Source: CAD feature listing. Evaluate the final solid. Frame: model axes, mm. Round coordinates to 2 decimals unless told otherwise and drop trailing zeros. Write each loop counter-clockwise with the first axis right and the second up, starting at its lowest first coordinate (ties: lowest second). Pieces come first, ordered by that corner, then holes.
from build123d import *

# Parameters (mm, degrees)
BOSS_EXTRUDE1_DEPTH = 5
FILLET1_R           = 8
SKETCH2_R           = 12.5
CUT_EXTRUDE1_DEPTH  = 10


with BuildPart() as part:
    # Sketch1 → Boss-Extrude1 (new body)
    with BuildSketch(Plane(origin=(0, 0, 0), x_dir=(1, 0, 0), z_dir=(0, 1, 0))):
        Polygon((-75.055534995, 0), (-37.527767497, -65), (37.527767497, -65), (75.055534995, 0), (37.527767497, 65), (-37.527767497, 65), align=None)
    extrude(amount=BOSS_EXTRUDE1_DEPTH)

    # Fillet1
    fillet1_edges = [part.edges().sort_by_distance(p)[0] for p in [
        (-37.527767497, 2.5, -65),
        (37.527767497, 2.5, -65),
        (75.055534995, 2.5, 0),
        (37.527767497, 2.5, 65),
        (-37.527767497, 2.5, 65),
        (-75.055534995, 2.5, 0),
    ]]
    fillet(fillet1_edges, radius=FILLET1_R)

    # Sketch2 → Cut-Extrude1 (cut)
    with BuildSketch(Plane(origin=(0, 5, 0), x_dir=(1, 0, 0), z_dir=(0, 1, 0))):
        with Locations(Location((0, 0, 0), (0, 0, 270))):
            Circle(SKETCH2_R)
        with BuildLine():
            Line((9.526279442, 26.5), (24.248711306, 52))
            ThreePointArc((24.248711306, 52), (24.248711306, 54), (22.516660498, 55))
            Line((22.516660498, 55), (-22.516660498, 55))
            ThreePointArc((-22.516660498, 55), (-24.248711306, 54), (-24.248711306, 52))
            Line((-24.248711306, 52), (-9.526279442, 26.5))
            ThreePointArc((-9.526279442, 26.5), (-8.42820323, 25.401923789), (-6.92820323, 25))
            Line((-6.92820323, 25), (6.92820323, 25))
            ThreePointArc((6.92820323, 25), (8.42820323, 25.401923789), (9.526279442, 26.5))
        make_face()
        with BuildLine():
            Line((27.712812921, 5), (57.15767665, 5))
            ThreePointArc((57.15767665, 5), (58.889727457, 6), (58.889727457, 8))
            Line((58.889727457, 8), (36.373066959, 47))
            ThreePointArc((36.373066959, 47), (34.641016151, 48), (32.908965344, 47))
            Line((32.908965344, 47), (18.186533479, 21.5))
            ThreePointArc((18.186533479, 21.5), (17.784609691, 20), (18.186533479, 18.5))
            Line((18.186533479, 18.5), (25.11473671, 6.5))
            ThreePointArc((25.11473671, 6.5), (26.212812921, 5.401923789), (27.712812921, 5))
        make_face()
        with BuildLine():
            Line((18.186533479, -21.5), (32.908965344, -47))
            ThreePointArc((32.908965344, -47), (34.641016151, -48), (36.373066959, -47))
            Line((36.373066959, -47), (58.889727457, -8))
            ThreePointArc((58.889727457, -8), (58.889727457, -6), (57.15767665, -5))
            Line((57.15767665, -5), (27.712812921, -5))
            ThreePointArc((27.712812921, -5), (26.212812921, -5.401923789), (25.11473671, -6.5))
            Line((25.11473671, -6.5), (18.186533479, -18.5))
            ThreePointArc((18.186533479, -18.5), (17.784609691, -20), (18.186533479, -21.5))
        make_face()
        with BuildLine():
            Line((-9.526279442, -26.5), (-24.248711306, -52))
            ThreePointArc((-24.248711306, -52), (-24.248711306, -54), (-22.516660498, -55))
            Line((-22.516660498, -55), (22.516660498, -55))
            ThreePointArc((22.516660498, -55), (24.248711306, -54), (24.248711306, -52))
            Line((24.248711306, -52), (9.526279442, -26.5))
            ThreePointArc((9.526279442, -26.5), (8.42820323, -25.401923789), (6.92820323, -25))
            Line((6.92820323, -25), (-6.92820323, -25))
            ThreePointArc((-6.92820323, -25), (-8.42820323, -25.401923789), (-9.526279442, -26.5))
        make_face()
        with BuildLine():
            Line((-27.712812921, -5), (-57.15767665, -5))
            ThreePointArc((-57.15767665, -5), (-58.889727457, -6), (-58.889727457, -8))
            Line((-58.889727457, -8), (-36.373066959, -47))
            ThreePointArc((-36.373066959, -47), (-34.641016151, -48), (-32.908965344, -47))
            Line((-32.908965344, -47), (-18.186533479, -21.5))
            ThreePointArc((-18.186533479, -21.5), (-17.784609691, -20), (-18.186533479, -18.5))
            Line((-18.186533479, -18.5), (-25.11473671, -6.5))
            ThreePointArc((-25.11473671, -6.5), (-26.212812921, -5.401923789), (-27.712812921, -5))
        make_face()
        with BuildLine():
            Line((-18.186533479, 21.5), (-32.908965344, 47))
            ThreePointArc((-32.908965344, 47), (-34.641016151, 48), (-36.373066959, 47))
            Line((-36.373066959, 47), (-58.889727457, 8))
            ThreePointArc((-58.889727457, 8), (-58.889727457, 6), (-57.15767665, 5))
            Line((-57.15767665, 5), (-27.712812921, 5))
            ThreePointArc((-27.712812921, 5), (-26.212812921, 5.401923789), (-25.11473671, 6.5))
            Line((-25.11473671, 6.5), (-18.186533479, 18.5))
            ThreePointArc((-18.186533479, 18.5), (-17.784609691, 20), (-18.186533479, 21.5))
        make_face()
    extrude(amount=-CUT_EXTRUDE1_DEPTH, mode=Mode.SUBTRACT)


solid = part.part
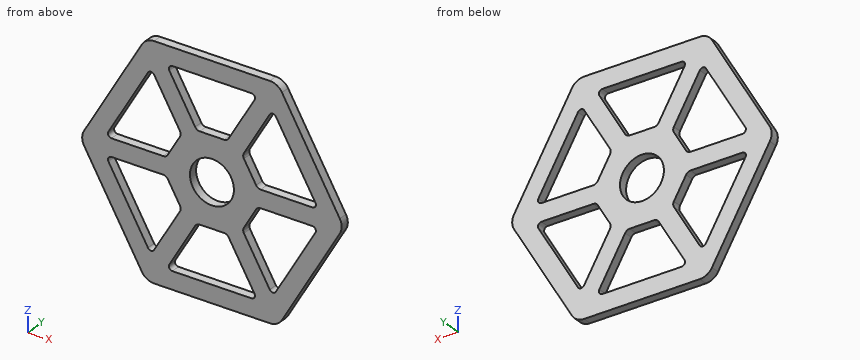
1) Section query C-C on z = 31. Return the cut outline in (x, y), then the cut area to 3 significant figures.
Taken from the geometry:
outline: (-57.16, 0) - (-45.61, 0) - (-45.61, 5) - (-57.16, 5) - close; (-23.67, 0) - (-12.12, 0) - (-12.12, 5) - (-23.67, 5) - close; (12.12, 0) - (23.67, 0) - (23.67, 5) - (12.12, 5) - close; (45.61, 0) - (57.16, 0) - (57.16, 5) - (45.61, 5) - close
area: 231 mm2
2) Section query D-D on y = 1.15. State how many separate pieces and enclosed holes the cut face has, then the cut area to 3 significant figures.
Taken from the geometry:
separate pieces: 1
enclosed holes: 7
area: 7,930 mm2
3) Section query B-B on z = 0. Return the cut outline in (x, y).
Taken from the geometry:
outline: (-73.82, 0) - (-12.5, 0) - (-12.5, 5) - (-73.82, 5) - close; (12.5, 0) - (73.82, 0) - (73.82, 5) - (12.5, 5) - close
4) Contact query for flat-ended pins moving along their axis: P1, Ø2.5, axis at x = 49.5, y = 3, coming from the -Z side; P2, Ø15, axis at x = 0, z = 0, coming from the -Y side. Output: stop coordinate, or through.
Taken from the geometry:
P1: stops at z = -46.43
P2: passes through
5) Material intervals for line 1 (X direction, y = 3.7, z = 0); line 2 (X direction, y = 1.05, z = 11); line 3 (X direction, y = 2.85, z = 29), sorted ascending.
Taken from the geometry:
line 1: x = -73.82 to -12.5, 12.5 to 73.82
line 2: x = -68.7 to -57.16, -22.52 to -5.94, 5.94 to 22.52, 57.16 to 68.7
line 3: x = -58.31 to -46.77, -22.52 to -10.97, 10.97 to 22.52, 46.77 to 58.31
6) Section query A-A on x = 0. Return the cut outline in (y, z).
Taken from the geometry:
outline: (0, -65) - (5, -65) - (5, -55) - (0, -55) - close; (0, -25) - (5, -25) - (5, -12.5) - (0, -12.5) - close; (0, 12.5) - (5, 12.5) - (5, 25) - (0, 25) - close; (0, 55) - (5, 55) - (5, 65) - (0, 65) - close
